Source: CAD feature listing. Evaluate the final solid. Frame: model axes, mm. Face numbers are marked on the shaded views. A direction names the side the tool comes from. Coordinates: 2 decimals unless noted, no trailing zeros. Write each loop counter-clockwise with the first axis right and the second up, starting at its lowest first coordinate (ties: lowest second). Pieces come first, ordered by that corner, then holes. Notation, with made-up numbers: (84, -36) -> (112, -36) arc R17 ccw to (112, -16) -> close; hole circle Ø11 at (32.5, -3.5). An arc over 180 degrees is marked (long way). One line per item, written item: value. Start each with the question number.
1. Mould query, pull axis X, two halves, no side actions, for the marked faces 5, 6 and 7. Classes: released by +X, released by -X, zero draft, split by the parting line, or undercut.
2. Access query for the marked faces 1, 2, 3 and 4. Directions: +Z, -Z, +X, -X, +Y, -Y. A direction counts if a zero-diameter tool reaches every point of the face in a straight line with its end or side. Return the directions, or none.
3. Section query B-B, the plane y = 93. Output: boundary loops of the cut face in (x, z), and give its area (3 significant figures).
4. Section query A-A, the plane x = 10. Output: boundary loops of the cut face in (y, z).
5. Line query: line 1 (Y direction, x = -15.5, z = 0); line 2 (X direction, y = 58.5, z = 0); line 3 (Y direction, x = 13.5, z = 2.25). Output: solid intervals per line, ascending.
6. Section query D-D, the plane z = 4.5. Output: boundary loops of the cut face in (x, y).
7. First-contact query: P1, Ø24, axis at x = -1.5, y = 91.5, coming from the -Z side; P2, Ø4.5, axis at y = 12, z = 0, coming from the -X side; P3, Ø8, axis at y = 102, z = 0, coming from the -X side; P4, Ø8, axis at y = 91, z = -2.5, coming from the +X side. Flat tips, straight axial feed; report the tip coordinate or a pass-through.
8. Section query C-C, the plane y = 10.5. Output: boundary loops of the cut face in (x, z).
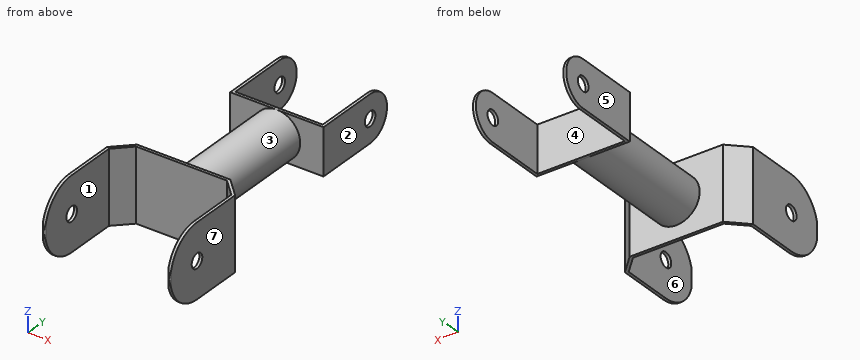
from build123d import *

# Parameters (mm, degrees)
BOSS_EXTRUDE1_DEPTH     = 12.5
BOSS_EXTRUDE1_2_DEPTH   = 12.5
CUT_EXTRUDE1_DEPTH      = 120.593059999
CUT_EXTRUDE1_DEPTH_BACK = 120.593059999
SKETCH3_R               = 2.5
SKETCH4_R               = 8
SKETCH4_R_2             = 6.000365116
BOSS_EXTRUDE2_DEPTH     = 44


with BuildPart() as part:
    # Sketch1 → Boss-Extrude1 (new, symmetric)
    with BuildSketch(Plane.XY):
        with BuildLine():
            Line((-16, 110), (-16, 80))
            Line((-16, 80), (16, 80))
            Line((16, 80), (16, 110))
            ThreePointArc((16, 110), (15.5, 110.5), (15, 110))
            Line((15, 110), (15, 81))
            Line((15, 81), (-15, 81))
            Line((-15, 81), (-15, 110))
            ThreePointArc((-15, 110), (-15.5, 110.5), (-16, 110))
        make_face()
    extrude(amount=BOSS_EXTRUDE1_DEPTH, both=True)


with BuildPart() as body_2:
    # Sketch1 → Boss-Extrude1 2 (new, symmetric)
    with BuildSketch(Plane.XY):
        with BuildLine():
            Line((-22, 0), (-22, 30))
            Line((-22, 30), (-16, 36))
            Line((-16, 36), (16, 36))
            Line((16, 36), (22, 30))
            Line((22, 30), (22, 0))
            ThreePointArc((22, 0), (21.5, -0.5), (21, 0))
            Line((21, 0), (21, 29.585786438))
            Line((21, 29.585786438), (15.585786438, 35))
            Line((15.585786438, 35), (-15.585786438, 35))
            Line((-15.585786438, 35), (-21, 29.585786438))
            Line((-21, 29.585786438), (-21, 0))
            ThreePointArc((-21, 0), (-21.5, -0.5), (-22, 0))
        make_face()
    extrude(amount=BOSS_EXTRUDE1_2_DEPTH, both=True)


with BuildPart() as cut_extrude1_tool:
    # Sketch3 → Cut-Extrude1 (new, two sides: drawn at the far end of the back side and taken through both)
    with BuildSketch(Plane(origin=(22, 0, 0), x_dir=(0, 0, -1), z_dir=(1, 0, 0)).offset(-CUT_EXTRUDE1_DEPTH_BACK)):
        with Locations(Location((0, 102, 0), (0, 0, 90))):
            Circle(SKETCH3_R)
        with Locations((0, 12)):
            Circle(SKETCH3_R)
        with BuildLine():
            Line((8, 80), (8, 102))
            ThreePointArc((8, 102), (0, 110), (-8, 102))
            Line((-8, 102), (-8, 80))
            Line((-8, 80), (-12.5, 80))
            Line((-12.5, 80), (-12.5, 110.5))
            Line((-12.5, 110.5), (12.5, 110.5))
            Line((12.5, 110.5), (12.5, 80))
            Line((12.5, 80), (8, 80))
        make_face()
        with BuildLine():
            Line((-12.5, 12), (-12.5, 36))
            Line((-12.5, 36), (-17.5, 36))
            Line((-17.5, 36), (-17.5, -4))
            Line((-17.5, -4), (17.5, -4))
            Line((17.5, -4), (17.5, 36))
            Line((17.5, 36), (12.5, 36))
            Line((12.5, 36), (12.5, 12))
            ThreePointArc((12.5, 12), (0, -0.5), (-12.5, 12))
        make_face()
    extrude(amount=CUT_EXTRUDE1_DEPTH + CUT_EXTRUDE1_DEPTH_BACK)


with BuildPart() as part_1:
    add(part.part)

    # Cut-Extrude1: cut by cut_extrude1_tool
    add(cut_extrude1_tool.part, mode=Mode.SUBTRACT)



with BuildPart() as body_2_1:
    add(body_2.part)

    # Cut-Extrude1: cut by cut_extrude1_tool
    add(cut_extrude1_tool.part, mode=Mode.SUBTRACT)


with BuildPart() as part_2:
    add(part_1.part)

    add(body_2_1.part)  # Boss-Extrude2 merges body 2
    # Sketch4 → Boss-Extrude2 (add)
    with BuildSketch(Plane(origin=(0, 36, 0), x_dir=(1, 0, 0), z_dir=(0, 1, 0))):
        with Locations(Location((0, 0, 0), (0, 0, 270))):
            Circle(SKETCH4_R)
        with Locations(Location((0, 0, 0), (0, 0, 270))):
            Circle(SKETCH4_R_2, mode=Mode.SUBTRACT)
    extrude(amount=BOSS_EXTRUDE2_DEPTH)


solid = part_2.part
Computed values:
1. face 5: released by -X
1. face 6: undercut
1. face 7: released by +X
2. face 1: +Z, -Z, -Y
2. face 2: +Z, -Z, +X, +Y
2. face 3: none
2. face 4: +Z, -Z, +Y
3. outline: (-16, -8) -> (-15, -8) -> (-15, 8) -> (-16, 8) -> close; (15, -8) -> (16, -8) -> (16, 8) -> (15, 8) -> close
3. area: 32.0 mm²
4. outline: (35, -12.5) -> (36, -12.5) -> (36, 12.5) -> (35, 12.5) -> close; (80, -8) -> (81, -8) -> (81, 8) -> (80, 8) -> close
5. line 1: y = 35 to 36, 80 to 99.5, 104.5 to 110
5. line 2: x = -8 to -6, 6 to 8
5. line 3: y = 35 to 36, 80 to 81
6. outline: (-22, 0.34) -> (-21, 0.34) -> (-21, 29.59) -> (-15.59, 35) -> (15.59, 35) -> (21, 29.59) -> (21, 0.34) -> (22, 0.34) -> (22, 30) -> (16, 36) -> (6.61, 36) -> (6.61, 80) -> (16, 80) -> (16, 108.61) -> (15, 108.61) -> (15, 81) -> (-15, 81) -> (-15, 108.61) -> (-16, 108.61) -> (-16, 80) -> (-6.61, 80) -> (-6.61, 36) -> (-16, 36) -> (-22, 30) -> close; hole (-3.97, 36) -> (3.97, 36) -> (3.97, 80) -> (-3.97, 80) -> close
7. P1: stops at z = -8
7. P2: passes through
7. P3: stops at x = -16
7. P4: stops at x = 16
8. outline: (-22, -12.41) -> (-21, -12.41) -> (-21, -2) -> (-22, -2) -> close; (-22, 2) -> (-21, 2) -> (-21, 12.41) -> (-22, 12.41) -> close; (21, -12.41) -> (22, -12.41) -> (22, -2) -> (21, -2) -> close; (21, 2) -> (22, 2) -> (22, 12.41) -> (21, 12.41) -> close
